Autodesk Inventor part; units mm, degrees
ref_plane "作業平面1" through (50.5, 0, 0) normal (1, 0, 0) x (0, 1, 0)
ref_plane "作業平面2" through (-50.5, 0, 0) normal (1, 0, 0) x (0, 1, 0)
ref_plane "作業平面3" through (0, 50.5, 0) normal (0, 1, 0) x (-1, 0, 0)
sketch "スケッチ1" plane through (0, 0, 0) normal (0, 0, 1) x (1, 0, 0)
  circle A0 centre (0, 0) radius 50.5
  dimension "d0" = 101
extrude "押し出し1" add sketch "スケッチ1" along normal blind 8
sketch "スケッチ2" plane through (0, 0, 8) normal (0, 0, 1) x (1, 0, 0)
  line L0 (-5, -5) -> (5, -5) construction
  line L1 (5, -5) -> (5, 5) construction
  line L2 (5, 5) -> (-5, 5) construction
  line L3 (-5, 5) -> (-5, -5) construction
  line L4 (-5, -5) -> (5, 5) construction
  line L5 (5, -5) -> (-5, 5) construction
  circle A0 centre (-5, 5) radius 1
  circle A1 centre (5, 5) radius 1
  circle A2 centre (5, -5) radius 1
  circle A3 centre (-5, -5) radius 1
  point P0 (0, 0)
  dimension "d3" = 10
  dimension "d4" = 10
  dimension "d5" = 2
  dimension "d6" = 2
  dimension "d7" = 2
  dimension "d8" = 2
extrude "押し出し2" cut sketch "スケッチ2" against normal blind 8
ref_plane "作業平面1" through (50.5, 0, 0) normal (1, 0, 0) x (0, 1, 0)
ref_plane "作業平面2" through (-50.5, 0, 0) normal (1, 0, 0) x (0, 1, 0)
ref_plane "作業平面3" through (0, 50.5, 0) normal (0, 1, 0) x (-1, 0, 0)
ref_plane "作業平面4" through (0, -50.5, 0) normal (0, 1, 0) x (-1, 0, 0)
sketch "スケッチ3" plane through (50.5, 0, 0) normal (1, 0, 0) x (0, 1, 0)
  line L0 (0, 0) -> (0, 4) construction
  circle A0 centre (0, 4) radius 1.5
  dimension "d14" = 4
  dimension "d15" = 3
extrude "押し出し3" cut sketch "スケッチ3" against normal blind 5
sketch "スケッチ4" plane through (-50.5, 0, 0) normal (1, 0, 0) x (0, 1, 0)
  line L0 (0, 0) -> (0, 4) construction
  circle A0 centre (0, 4) radius 1.5
  dimension "d18" = 4
  dimension "d19" = 3
extrude "押し出し4" cut sketch "スケッチ4" along normal blind 5
sketch "スケッチ5" plane through (0, 50.5, 0) normal (0, 1, 0) x (-1, 0, 0)
  line L0 (0, 0) -> (0, 4) construction
  circle A0 centre (0, 4) radius 1.5
  dimension "d22" = 4
  dimension "d23" = 3
extrude "押し出し5" cut sketch "スケッチ5" against normal blind 5
sketch "スケッチ6" plane through (0, -50.5, 0) normal (0, 1, 0) x (-1, 0, 0)
  line L0 (0, 0) -> (0, 4) construction
  circle A0 centre (0, 4) radius 1.5
  dimension "d26" = 4
  dimension "d27" = 3
extrude "押し出し6" cut sketch "スケッチ6" along normal blind 5
thread "ねじ1"
thread "ねじ2"
thread "ねじ3"
thread "ねじ4"
thread "ねじ5"
thread "ねじ6"
thread "ねじ7"
thread "ねじ8"
properties part number "outsideBottom2"
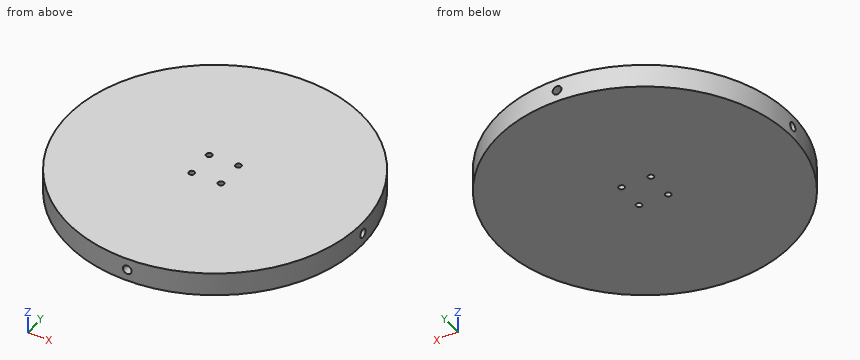
CAD build for the part. Positions are in the model's coordinates, mm. Give positions to 0.01 mm unless a question says otherwise; leave off trailing zeros. Order: outer loops, then holes, each group sorted by start corner. A loop starts at its lowest first (then second) coordinate and runs counter-clockwise, first axis right, second up. Notation, with made-up numbers: (60.25, 27.5) -> (119.25, 27.5) arc R9 cw to (119.25, 37.5) -> close; hole circle Ø4 at (18.25, 29.25). An arc over 180 degrees is marked (long way). Return JSON: item names as keys, results as strings.
Q1. Flat gauge pins, fed straight in: pin 1 (1 mm diameter, centred on y = -19.5, z = 4, fed in from +X); pin 2 (2.5 mm diameter, centred on y = 0, z = 4, fed in from +X); pin 3 (1.5 mm diameter, centred on x = 2.5, z = 3.5, fed in from -Y). Where does each tip first touch, or does it go through?
Working result:
{"pin 1": "x = 46.79", "pin 2": "x = 45.5", "pin 3": "y = -50.47"}
Q2. Saw through at A-A (z = 4). Write the cut outline in (x, y), then the cut area to 3 significant figures.
Working result:
{"outline": "(-50.48, -1.5) arc R50.5 ccw to (-1.5, -50.48) -> (-1.5, -45.5) -> (1.5, -45.5) -> (1.5, -50.48) arc R50.5 ccw to (50.48, -1.5) -> (45.5, -1.5) -> (45.5, 1.5) -> (50.48, 1.5) arc R50.5 ccw to (1.5, 50.48) -> (1.5, 45.5) -> (-1.5, 45.5) -> (-1.5, 50.48) arc R50.5 ccw to (-50.48, 1.5) -> (-45.5, 1.5) -> (-45.5, -1.5) -> close; hole circle Ø2 at (-5, -5); hole circle Ø2 at (-5, 5); hole circle Ø2 at (5, -5); hole circle Ø2 at (5, 5)", "area": "7,940 mm²"}
Q3. Saw through at D-D (x = -14.5). Write the cut outline in (y, z), then the cut area to 3 significant figures.
Working result:
{"outline": "(-48.37, 0) -> (48.37, 0) -> (48.37, 8) -> (-48.37, 8) -> close", "area": "774 mm²"}
Q4. Saw through at B-B (x = 0). Write the cut outline in (y, z).
Working result:
{"outline": "(-50.5, 0) -> (50.5, 0) -> (50.5, 2.5) -> (45.5, 2.5) -> (45.5, 5.5) -> (50.5, 5.5) -> (50.5, 8) -> (-50.5, 8) -> (-50.5, 5.5) -> (-45.5, 5.5) -> (-45.5, 2.5) -> (-50.5, 2.5) -> close"}
Q5. Drill centre lines: line 1 (Z direction, x = 0, y = 47.15); line 2 (X direction, y = 1.5, z = 5.5); line 3 (X direction, y = 42.5, z = 3.25). Where is each one in solid material? Low to high.
Working result:
{"line 1": "0 to 2.5, 5.5 to 8", "line 2": "-50.48 to 50.48", "line 3": "-27.28 to 27.28"}
